from build123d import *

# Parameters (mm, degrees)
F0_R     = 76.2
F1_DEPTH = 533.4


with BuildPart() as f1:
    # F0 (on Front) → F1 (new body)
    with BuildSketch(Plane.XZ):
        Circle(F0_R)
        with BuildLine():
            ThreePointArc((2.540587, 25.272622), (-0.000565, -25.4), (-2.539463, 25.272735))
            Line((-2.539463, 25.272735), (-2.495172, 15.24))
            Line((-2.495172, 15.24), (2.584878, 15.24))
            Line((2.584878, 15.24), (2.540587, 25.272622))
        make_face(mode=Mode.SUBTRACT)
    extrude(amount=F1_DEPTH)

    # F2 (on Top) → F3 (revolve, cut)
    with BuildSketch(Plane.XY):
        Polygon((-50.8, -50.8), (-50.8, 0), (-89.3064, 0), (-89.3064, -127), (-89.3064, -203.2), (-89.3064, -330.2), (-86.315122, -406.4), (-86.315122, -533.4), (-48.215122, -533.4), (-48.215122, -482.6), (-73.615122, -482.6), (-73.615122, -457.2), (-48.215122, -457.2), (-48.215122, -406.4), (-35.515122, -406.4), (-35.515122, -330.2), (-48.215122, -330.2), (-48.215122, -279.4), (-73.615122, -279.4), (-73.615122, -254), (-48.215122, -254), (-48.215122, -203.2), (-35.515122, -203.2), (-35.515122, -127), (-50.8, -127), (-50.8, -76.2), (-76.2, -76.2), (-76.2, -50.8), align=None)
    revolve(axis=Axis((2.584878, -165.1, 0), (0, -1, 0)), mode=Mode.SUBTRACT)


solid = f1.part
Work out the finished part from the listing and answer in its coordinate system (mm). A direction names the side the tool comes from. Round coordinates to 2 decimals unless told otherwise and drop trailing zeros. Write each loop counter-clockwise with the first axis right and the second up, starting at its lowest first coordinate (ties: lowest second). Pieces come first, ordered by that corner, then holes. Notation, with made-up numbers: (63.5, -37.75) - (106.5, -37.75) arc R12 ccw to (106.5, -14.75) - close; hole circle Ø3 at (-24.75, 81). An arc over 180 degrees is marked (long way). Answer in a Markdown table with one row per item. Add a question column.
1. Find the intervals of material crossed by line 1 along Y through (x, z) = (24.5, -66); line 2 along Y through (x, z) = (40, 20); line 3 along Z through (x, y) = (0, -395), in increasing order. Write a range as from..to.
2. Given pin 1 (4 mm diameter, centred on x = 1, y = -354, fed in from -Z); pin 2 (6 mm diameter, centred on x = -51.5, z = 39, fed in from -Y); pin 3 (2 mm diameter, centred on y = -409, z = 53, fed in from +X); pin 4 (2 mm diameter, centred on y = -127.5, z = 4.5, fed in from -X), each flat-ended and moving along its own axis, determine where each tip first touches the part or whether it passes through.
3. For faces 1 (the flat face through (-5, -406.4, -38)), 2 (the flat face through (24, -533.4, -11)), 3 (the flat face through (-50, -50.8, 16)), determine the directions among +Z, -Z, +X, -X, +Y, -Y from which every point of the face is accessible in a straight line to the end or side of a thin tool.
4. A cutting plane is placed at C-C, the plane z = 65. Determine the outline of the cut face in (x, y).
5. A cutting plane is placed at A-A, the plane y = -436.5. Determine the outline of the cut face in (x, z).
6. A cutting plane is placed at B-B, the plane z = -60. Determine the outline of the cut face in (x, y), and give its area (3 significant figures).
Worked out:
| question | item | result |
|---|---|---|
| 1 | line 1 | -482.6..-457.2, -279.4..-254, -76.2..-50.8 |
| 1 | line 2 | -533.4..-406.4, -330.2..-203.2, -127..0 |
| 1 | line 3 | -38.01..-25.4, 15.24..38.01 |
| 2 | pin 1 | z = -38.1 |
| 2 | pin 2 | y = -482.6 |
| 2 | pin 3 | through |
| 2 | pin 4 | x = -50.68 |
| 3 | face 1 | none |
| 3 | face 2 | +Z, -Z, +X, -X, -Y |
| 3 | face 3 | +Y |
| 4 | outline | (-39.77, -76.2) - (39.77, -76.2) - (39.77, -50.8) - (-39.77, -50.8) - close; (-37.18, -482.6) - (39.77, -482.6) - (39.77, -457.2) - (-37.18, -457.2) - close; (-37.18, -279.4) - (39.77, -279.4) - (39.77, -254) - (-37.18, -254) - close |
| 5 | outline | circle Ø101.6 at (2.58, 0); hole (-2.54, 25.27) arc R25.4 ccw (long way) to (2.54, 25.27) - (2.58, 15.24) - (-2.5, 15.24) - close |
| 6 | outline | (-46.97, -76.2) - (46.97, -76.2) - (46.97, -50.8) - (-46.97, -50.8) - close; (-44.39, -482.6) - (46.97, -482.6) - (46.97, -457.2) - (-44.39, -457.2) - close; (-44.39, -279.4) - (46.97, -279.4) - (46.97, -254) - (-44.39, -254) - close |
| 6 | area | 7,030 mm^2 |
